Can you work these out from the model? Positions are in its coordinate system, mm. A direction names the side the tool comes from. Round coordinates to 2 decimals unless told otherwise and drop trailing zeros. Loops run counter-clockwise (first coordinate to the right, second up) from the corner with the lowest first, then second, coordinate; pieces in that order, holes last. Notation, with made-up numbers: (-24.75, 37) -> (24.25, 37) arc R21 cw to (24.25, 59) -> close; hole circle Ø8 at (9, 23). An arc over 180 degrees is marked (long way). Answer as a JSON object with one key per item and string values.
```python
from build123d import *

# Parameters (mm, degrees)
SKETCH_1_W          = 110
SKETCH_1_H          = 21
EXTRUDE_1_DEPTH     = 20
CUT_EXTRUDE_1_REACH = 115.759
SKETCH_2_R          = 2.15
CUT_EXTRUDE_2_REACH = 115.759
SKETCH_3_W          = 60
SKETCH_3_H          = 6
FILLET_2_R          = 2


with BuildPart() as part:
    # 草图1 → 凸台-拉伸1 (new body)
    with BuildSketch(Plane.XY):
        with Locations((-55, 10.5)):
            Rectangle(SKETCH_1_W, SKETCH_1_H)
    extrude(amount=EXTRUDE_1_DEPTH)

    # 草图2 → 切除-拉伸1 (cut, up to next)
    with BuildSketch(Plane(origin=(0, 21, 0), x_dir=(1, 0, 0), z_dir=(0, 1, 0)), mode=Mode.PRIVATE) as cut_extrude_1_sk1:
        with Locations(Location((-15, -10, 0), (0, 0, 180))):
            Circle(SKETCH_2_R)
    cut_extrude_1_tool1 = extrude(cut_extrude_1_sk1.sketch, amount=-CUT_EXTRUDE_1_REACH, mode=Mode.PRIVATE) & part.part
    # 草图2 → 切除-拉伸1 (cut, up to next)
    with BuildSketch(Plane(origin=(0, 21, 0), x_dir=(1, 0, 0), z_dir=(0, 1, 0)), mode=Mode.PRIVATE) as cut_extrude_1_sk2:
        with Locations(Location((-5, -10, 0), (0, 0, 180))):
            Circle(SKETCH_2_R)
    cut_extrude_1_tool2 = extrude(cut_extrude_1_sk2.sketch, amount=-CUT_EXTRUDE_1_REACH, mode=Mode.PRIVATE) & part.part
    # 草图2 → 切除-拉伸1 (cut, up to next)
    with BuildSketch(Plane(origin=(0, 21, 0), x_dir=(1, 0, 0), z_dir=(0, 1, 0)), mode=Mode.PRIVATE) as cut_extrude_1_sk3:
        with Locations(Location((-105, -10, 0), (0, 0, 180))):
            Circle(SKETCH_2_R)
    cut_extrude_1_tool3 = extrude(cut_extrude_1_sk3.sketch, amount=-CUT_EXTRUDE_1_REACH, mode=Mode.PRIVATE) & part.part
    # 草图2 → 切除-拉伸1 (cut, up to next)
    with BuildSketch(Plane(origin=(0, 21, 0), x_dir=(1, 0, 0), z_dir=(0, 1, 0)), mode=Mode.PRIVATE) as cut_extrude_1_sk4:
        with Locations(Location((-95, -10, 0), (0, 0, 180))):
            Circle(SKETCH_2_R)
    cut_extrude_1_tool4 = extrude(cut_extrude_1_sk4.sketch, amount=-CUT_EXTRUDE_1_REACH, mode=Mode.PRIVATE) & part.part
    add(cut_extrude_1_tool1.solids().sort_by_distance((-15, 21, 10))[0], mode=Mode.SUBTRACT)
    add(cut_extrude_1_tool2.solids().sort_by_distance((-5, 21, 10))[0], mode=Mode.SUBTRACT)
    add(cut_extrude_1_tool3.solids().sort_by_distance((-105, 21, 10))[0], mode=Mode.SUBTRACT)
    add(cut_extrude_1_tool4.solids().sort_by_distance((-95, 21, 10))[0], mode=Mode.SUBTRACT)

    # 草图3 → 切除-拉伸2 (cut, up to next)
    with BuildSketch(Plane(origin=(0, 21, 0), x_dir=(1, 0, 0), z_dir=(0, 1, 0)), mode=Mode.PRIVATE) as cut_extrude_2_sk1:
        with Locations((-55, -3)):
            Rectangle(SKETCH_3_W, SKETCH_3_H)
    cut_extrude_2_tool1 = extrude(cut_extrude_2_sk1.sketch, amount=-CUT_EXTRUDE_2_REACH, mode=Mode.PRIVATE) & part.part
    # 草图3 → 切除-拉伸2 (cut, up to next)
    with BuildSketch(Plane(origin=(0, 21, 0), x_dir=(1, 0, 0), z_dir=(0, 1, 0)), mode=Mode.PRIVATE) as cut_extrude_2_sk2:
        with Locations((-55, -17)):
            Rectangle(SKETCH_3_W, SKETCH_3_H)
    cut_extrude_2_tool2 = extrude(cut_extrude_2_sk2.sketch, amount=-CUT_EXTRUDE_2_REACH, mode=Mode.PRIVATE) & part.part
    add(cut_extrude_2_tool1.solids().sort_by_distance((-55, 21, 3))[0], mode=Mode.SUBTRACT)
    add(cut_extrude_2_tool2.solids().sort_by_distance((-55, 21, 17))[0], mode=Mode.SUBTRACT)

    # 圆角2
    fillet_2_edges = [part.edges().sort_by_distance(p)[0] for p in [
        (-110, 10.5, 20),
        (-97.5, 0, 20),
        (-12.5, 0, 0),
        (-97.5, 21, 0),
        (-97.5, 21, 20),
        (-12.5, 0, 20),
        (-85, 10.5, 6),
        (-85, 10.5, 0),
        (-25, 10.5, 0),
        (-25, 10.5, 6),
        (-85, 21, 3),
        (-55, 21, 6),
        (-25, 21, 3),
        (-55, 0, 6),
        (-85, 0, 3),
        (-25, 0, 3),
        (-25, 10.5, 20),
        (-85, 10.5, 20),
        (-85, 10.5, 14),
        (-25, 10.5, 14),
        (0, 10.5, 20),
        (-97.5, 0, 0),
        (-25, 21, 17),
        (-55, 21, 14),
        (-85, 21, 17),
        (-85, 0, 17),
        (-55, 0, 14),
        (-25, 0, 17),
        (-110, 10.5, 0),
        (-12.5, 21, 0),
        (0, 10.5, 0),
        (-12.5, 21, 20),
    ]]
    fillet(fillet_2_edges, radius=FILLET_2_R)


solid = part.part
```
Q1. I want a section at A-A, the plane x = -5. Write out the boundary of the cut face in (y, z).
Determined:
{"outline": "(0, 2) arc R2 ccw to (2, 0) -> (19, 0) arc R2 ccw to (21, 2) -> (21, 7.85) -> (0, 7.85) -> close; (0, 12.15) -> (21, 12.15) -> (21, 18) arc R2 ccw to (19, 20) -> (2, 20) arc R2 ccw to (0, 18) -> close"}
Q2. I want a section at C-C, the plane z = 10. Write out the boundary of the cut face in (x, y).
Determined:
{"outline": "(-110, 0) -> (-107.15, 0) -> (-107.15, 21) -> (-110, 21) -> close; (-102.85, 0) -> (-97.15, 0) -> (-97.15, 21) -> (-102.85, 21) -> close; (-92.85, 0) -> (-17.15, 0) -> (-17.15, 21) -> (-92.85, 21) -> close; (-12.85, 0) -> (-7.15, 0) -> (-7.15, 21) -> (-12.85, 21) -> close; (-2.85, 0) -> (0, 0) -> (0, 21) -> (-2.85, 21) -> close"}
Q3. I'm going to push flat-ended pins straight in: pin 1 (1.5 mm diameter, centred on x = -52.5, y = 11, fed in from +Z); pin 2 (6 mm diameter, centred on x = -31.5, z = 4.5, fed in from +Y). Where does each tip first touch, or does it pass through?
Determined:
{"pin 1": "z = 14", "pin 2": "y = 20.94"}
Q4. We'd pull the mould along Z, two halves only. Please class faces 6 (the cylindrical face through (-102.85, 10.65, 10.09)), 7 (the cylindrical face through (-11.34, 0.57, 0.6)), 8 (the flat face through (-13, 11, 20)): pulls with the +Z half, pulls with the -Z half, needs draft (parallel to the pull), parting line crosses it, or undercut.
Determined:
{"face 6": "undercut", "face 7": "pulls with the -Z half", "face 8": "pulls with the +Z half"}
Q5. On a 3-axis mill with a long thin cutter (end or side, diameter ignored), from which of +Z, -Z, +X, -X, +Y, -Y can I reach the whole of each face in a straight line? I mean faces 1 (the cylindrical face through (-11.34, 20.43, 19.4)), 2 (the cylindrical face through (-85.6, 20.43, 2.99)), 3 (the flat face through (-98, 11, 20)), 4 (the flat face through (-85, 11, 17)), 5 (the flat face through (-85, 11, 3)). Say none if no direction works.
Determined:
{"face 1": "+Z, +X, -X, +Y", "face 2": "-Z, +Y", "face 3": "+Z, +X, -X, +Y, -Y", "face 4": "+Z, +Y, -Y", "face 5": "-Z, +Y, -Y"}
Q6. I want a section at B-B, the plane y = 10.75. Write out the boundary of the cut face in (x, z).
Determined:
{"outline": "(-110, 2) arc R2 ccw to (-108, 0) -> (-87, 0) arc R2 ccw to (-85, 2) -> (-85, 4) arc R2 cw to (-83, 6) -> (-27, 6) arc R2 cw to (-25, 4) -> (-25, 2) arc R2 ccw to (-23, 0) -> (-2, 0) arc R2 ccw to (0, 2) -> (0, 18) arc R2 ccw to (-2, 20) -> (-23, 20) arc R2 ccw to (-25, 18) -> (-25, 16) arc R2 cw to (-27, 14) -> (-83, 14) arc R2 cw to (-85, 16) -> (-85, 18) arc R2 ccw to (-87, 20) -> (-108, 20) arc R2 ccw to (-110, 18) -> close; hole circle Ø4.3 at (-105, 10); hole circle Ø4.3 at (-95, 10); hole circle Ø4.3 at (-15, 10); hole circle Ø4.3 at (-5, 10)"}
Q7. If I drill on L1, parallel to Z at x = -105, y = 9; L2, parallel to X at y = 10.5, z = 1.75; L3, parallel to X at y = 9.5, z = 9.5, over which ranges is the centre line in solid material (lowest first)? Write a range as [from, to].
Determined:
{"L1": "[0, 7.85], [12.15, 20]", "L2": "[-109.98, -85.02], [-24.98, -0.02]", "L3": "[-110, -107.09], [-102.91, -97.09], [-92.91, -17.09], [-12.91, -7.09], [-2.91, 0]"}
Q8. I want a section at D-D, the plane x = -69.5. Write out the boundary of the cut face in (y, z), then the cut area to 3 significant figures.
Determined:
{"outline": "(0, 8) arc R2 ccw to (2, 6) -> (19, 6) arc R2 ccw to (21, 8) -> (21, 12) arc R2 ccw to (19, 14) -> (2, 14) arc R2 ccw to (0, 12) -> close", "area": "165 mm²"}
